Autodesk Inventor part; units mm, degrees
ref_plane "YZ Plane" through (0, 0, 0) normal (1, 0, 0) x (0, 1, 0)
ref_plane "XZ Plane" through (0, 0, 0) normal (0, 1, 0) x (-1, 0, 0)
ref_plane "XY Plane" through (0, 0, 0) normal (0, 0, 1) x (1, 0, 0)
sketch "Sketch1" plane through (0, 0, 0) normal (0, 0, 1) x (1, 0, 0)
  line L0 (-21.725, -10) -> (-22.225, -10) construction
  line L1 (-22.225, -10) -> (-22.225, 0) construction
  line L2 (-22.225, 0) -> (-21.725, 0) construction
  line L3 (-21.725, 0) -> (-21.725, -10) construction
  line L4 (-22, 37) -> (-19.3551, 22)
  line L5 (-22.5, 12) -> (-22.5, 24)
  line L6 (-22.5, 24) -> (-21.5, 24)
  line L7 (-21.5, 24) -> (-21.5, 26)
  line L8 (-21.5, 26) -> (-22.5, 26)
  line L9 (-22.5, 26) -> (-22.5, 37)
  line L10 (-22, 37) -> (-22.5, 37)
  line L11 (0, -19.4) -> (0, 46.4)
  line L12 (-20, 22) -> (-19.3551, 22)
  line L13 (-22.5, 12) -> (-21.725, 12)
  line L14 (-21.725, 12) -> (-21.725, 0)
  line L15 (-21.725, 0) -> (-20, 0)
  line L16 (-20, 0) -> (-20, 22)
  point P0 (0, 0)
  dimension "d0" = 10
  dimension "d1" = 22.225
  dimension "d3" = 0.5
  dimension "d5" = 11
  dimension "d6" = 2
  dimension "d7" = 22.5
  dimension "d12" = 1
  dimension "d18" = 0.5
  dimension "d19" = 10
  dimension "d20" = 15
  dimension "d21" = 12
  dimension "d22" = 37
  dimension "d24" = 20
revolve "Revolution1" add sketch "Sketch1" angle 360 about axis through (0, -10, 0) along (0, 1, 0)
properties part number "CapConeThin" material "Brass"
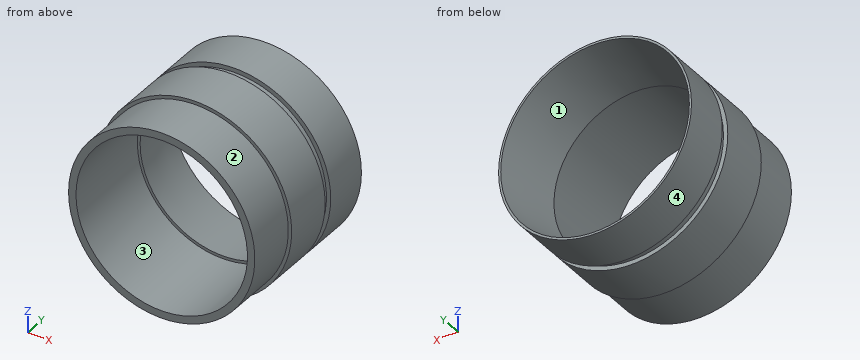
Build history of the part. All positions in model axes, mm. Face numbers are marked on the shaded views. A direction names the side the tool comes from. Round coordinates to 2 decimals unless told otherwise and drop trailing zeros. Write each loop counter-clockwise with the first axis right and the second up, starting at its lowest first coordinate (ties: lowest second). Pieces come first, ordered by that corner, then holes. Notation, with made-up numbers: (-22, 10.25) -> (-13, 10.25) arc R13 ccw to (-13, 14.25) -> close; hole circle Ø5 at (22.25, 61.25). An arc over 180 degrees is marked (long way). Put each result on its own line as item: value.
Item 1: Slice it at D-D, the plane y = 29.5. Give the cut face in (x, z), plus the area to 3 significant figures.
Here are the results:
outline: circle Ø45 at (0, 0); hole circle Ø41.36 at (0, 0)
area: 247 mm^2
Item 2: Flat gauge pins, fed straight in: P1, Ø8, axis at x = -6.5, y = 11, coming from the +Z side; P2, Ø10, axis at y = 27.5, z = 15, coming from the +X side; P3, Ø5, axis at x = 5.5, y = 10, coming from the -Z side. Where does each tip first touch, or does it go through?
Here are the results:
P1: stops at z = 22.35
P2: stops at x = 20.16
P3: stops at z = -22.14
Item 3: Wall check: probe 1 along Z at (x, y) = (0, 13.75); probe 2 along Z at (x, y) = (0, 8) (3 decimals); probe 3 along Y at (x, z) = (13, -18). Give the ranges that are in metal, low to high. Write a range as from..to.
Here are the results:
probe 1: z = -22.5..-20, 20..22.5
probe 2: z = -21.725..-20, 20..21.725
probe 3: y = 12..24, 26..37
Item 4: Two-plate mould, pull along X, no slides. Class the marked faces 1 and 2: pulls with the +X half, pulls with the -X half, needs draft (parallel to the pull), parting line crosses it, or undercut.
Here are the results:
face 1: undercut
face 2: parting line crosses it
Item 5: Slice it at B-B, the plane y = 5.5. Give the cut face in (x, z) (3 decimals), plus the area to 3 significant figures.
Here are the results:
outline: circle Ø43.45 at (0, 0); hole circle Ø40 at (0, 0)
area: 226 mm^2
Item 6: Tool access for the marked faces 3 and 4: list every direction of +Z, -Z, +X, -X, +Y, -Y with a clear straight run to the whole face (end or side of a thin tool).
Here are the results:
face 3: -Y
face 4: +Y, -Y
Item 7: Slice it at A-A, the plane z = 0. Give the cut face in (x, y) (3 decimals).
Here are the results:
outline: (-22.5, 12) -> (-21.725, 12) -> (-21.725, 0) -> (-20, 0) -> (-20, 22) -> (-19.355, 22) -> (-22, 37) -> (-22.5, 37) -> (-22.5, 26) -> (-21.5, 26) -> (-21.5, 24) -> (-22.5, 24) -> close; (19.355, 22) -> (20, 22) -> (20, 0) -> (21.725, 0) -> (21.725, 12) -> (22.5, 12) -> (22.5, 24) -> (21.5, 24) -> (21.5, 26) -> (22.5, 26) -> (22.5, 37) -> (22, 37) -> close
Item 8: Slice it at C-C, the plane x = 0. Give the cut face in (y, z) (3 decimals).
Here are the results:
outline: (0, -21.725) -> (12, -21.725) -> (12, -22.5) -> (24, -22.5) -> (24, -21.5) -> (26, -21.5) -> (26, -22.5) -> (37, -22.5) -> (37, -22) -> (22, -19.355) -> (22, -20) -> (0, -20) -> close; (0, 20) -> (22, 20) -> (22, 19.355) -> (37, 22) -> (37, 22.5) -> (26, 22.5) -> (26, 21.5) -> (24, 21.5) -> (24, 22.5) -> (12, 22.5) -> (12, 21.725) -> (0, 21.725) -> close
